```python
from build123d import *

# Parameters (mm, degrees)
SKETCH1_W                    = 42
SKETCH1_H                    = 42
SKETCH1_R                    = 1.65
SKETCH1_R_2                  = 18
BOSS_EXTRUDE1_DEPTH          = 13
CHAMFER1_SIZE                = 5.5
SKETCH3_R                    = 1.75
CUT_EXTRUDE2_DEPTH           = 20
SKETCH4_R                    = 1.75
CUT_EXTRUDE3_DEPTH           = 20
BOSS_EXTRUDE2_DEPTH          = 2
CUT_REVOLVE1_ANGLE           = 183.3
CUT_REVOLVE1_OTHER_WAY_ANGLE = 3.2


with BuildPart() as part:
    # Sketch1 → Boss-Extrude1 (new body)
    with BuildSketch(Plane(origin=(0, 0, 0), x_dir=(1, 0, 0), z_dir=(0, 1, 0))):
        with Locations((21, 21)):
            Rectangle(SKETCH1_W, SKETCH1_H)
        with Locations(Location((5.5, 36.5, 0), (0, 0, 90))):
            Circle(SKETCH1_R, mode=Mode.SUBTRACT)
        with Locations(Location((5.5, 5.5, 0), (0, 0, 90))):
            Circle(SKETCH1_R, mode=Mode.SUBTRACT)
        with Locations(Location((21, 21, 0), (0, 0, 90))):
            Circle(SKETCH1_R_2, mode=Mode.SUBTRACT)
    extrude(amount=BOSS_EXTRUDE1_DEPTH)

    # Chamfer1
    chamfer1_edges = [part.edges().sort_by_distance(p)[0] for p in [
        (0, 6.5, -42),
        (42, 6.5, -42),
        (42, 6.5, 0),
        (0, 6.5, 0),
    ]]
    chamfer(chamfer1_edges, length=CHAMFER1_SIZE)

    # Sketch3 → Cut-Extrude2 (cut)
    with BuildSketch(Plane(origin=(42, 0, 0), x_dir=(0, 0, -1), z_dir=(1, 0, 0))):
        with Locations(Location((37.4, 9, 0), (0, 0, 333.948601241))):
            Circle(SKETCH3_R)
    extrude(amount=-CUT_EXTRUDE2_DEPTH, mode=Mode.SUBTRACT)

    # Sketch4 → Cut-Extrude3 (cut)
    with BuildSketch(Plane(origin=(42, 0, 0), x_dir=(0, 0, -1), z_dir=(1, 0, 0))):
        with Locations(Location((4.6, 9, 0), (0, 0, 300.949723079))):
            Circle(SKETCH4_R)
    extrude(amount=-CUT_EXTRUDE3_DEPTH, mode=Mode.SUBTRACT)

    # Sketch6 → Boss-Extrude2 (add)
    with BuildSketch(Plane(origin=(0, 0, -42), x_dir=(-1, 0, 0), z_dir=(0, 0, -1))):
        Polygon((-23.468351512, 0.829629357), (-18.531648488, 0.829629357), (-18.531648488, 5.944922789), (-14.8, 5.944922789), (-21, 12.144922789), (-27.2, 5.944922789), (-23.468351512, 5.944922789), align=None)
    extrude(amount=BOSS_EXTRUDE2_DEPTH)

    # Sketch9 → Cut-Revolve1 (revolve, cut)
    with BuildSketch(Plane(origin=(21, 0, 0), x_dir=(0, 0, -1), z_dir=(1, 0, 0))):
        with BuildLine():
            Line((3.027799244, 9.768560202), (3.027799244, 8.231439798))
            ThreePointArc((3.027799244, 8.231439798), (2.85, 9), (3.027799244, 9.768560202))
        make_face()
    revolve(axis=Axis((21, 18.192178388, -21), (0, -1, 0)), revolution_arc=CUT_REVOLVE1_ANGLE, mode=Mode.SUBTRACT)

    # Sketch9 → Cut-Revolve1 other way (revolve, cut)
    with BuildSketch(Plane(origin=(21, 0, 0), x_dir=(0, 0, -1), z_dir=(1, 0, 0))):
        with BuildLine():
            Line((3.027799244, 9.768560202), (3.027799244, 8.231439798))
            ThreePointArc((3.027799244, 8.231439798), (2.85, 9), (3.027799244, 9.768560202))
        make_face()
    revolve(axis=Axis((21, 18.192178388, -21), (0, 1, 0)), revolution_arc=CUT_REVOLVE1_OTHER_WAY_ANGLE, mode=Mode.SUBTRACT)


solid = part.part
```
For this review, take the finished solid that the model builds, in its own axes (mm). A direction names the side the tool comes from. Give positions to 0.01 mm unless a question says otherwise; leave off trailing zeros. Write each loop counter-clockwise with the first axis right and the second up, starting at its lowest first coordinate (ties: lowest second). Pieces come first, ordered by that corner, then holes.
Item 1: Machinability: for faces 4 (the face through (24.057, 9.088, -42.986)), 5 (the face through (17.857, 9.002, -42.986)), 6 (the face through (34.36, 9.64, -2.97)), which of the approach directions +Z, -Z, +X, -X, +Y, -Y give a long, thin tool a straight path to every point of the face, cutting with its end or side? Answer none if there is none.
Item 2: Insertion check: P1, Ø1, axis at x = 21, z = -43, coming from the -Y side; P2, Ø1, axis at y = 3, z = -43.5, coming from the +X side; P3, Ø0.6, axis at x = 17.5, z = -43.5, coming from the -Y side; P4, Ø3, axis at x = 5.5, z = -5.5, coming from the +Y side. Each pin has a flat end and moves straight along its axis. Give the tip position at first contact, or say it passes through.
Item 3: Take a section at A-A (y = 9). Give the number of separate pieces and of enclosed holes in the cut face, and give its area (3 significant figures).
Item 4: Take a section at C-C (y = 1.75). Give the boundary of the cut face in (x, z), and give its area (3 significant figures).
Item 5: Take a section at D-D (x = 24). Give the boundary of the cut face in (y, z).
Item 6: Wall thickness on probe 1 along Z at (x, y) = (22, 3.75); probe 2 along X at (y, z) = (7, -36.5); probe 3 along Z at (x, y) = (36, 9): over which ranges is each line inside the solid? List them lowest first.
Item 7: The part is to be moulded in two halves that separate along X. For faces 1 (the face through (25, 5.945, -43)), 2 (the face through (23.468, 3, -43)), 3 (the face through (31.953, 6.409, -6.716)), say which applies: +X half, -X half, draft (parallel to the pull), parting line (faces both ways), or undercut.
Item 8: Take a section at B-B (z = -21). Give the boundary of the cut face in (x, y).
Established:
1. face 4: -Z, +X, +Y
1. face 5: -Z, -X, +Y
1. face 6: +X
2. P1: stops at y = 0.83
2. P2: stops at x = 23.47
2. P3: stops at y = 5.94
2. P4: passes through
3. separate pieces: 2
3. enclosed holes: 2
3. area: 580 mm2
4. outline: (0, -36.5) - (5.5, -42) - (18.53, -42) - (18.53, -44) - (23.47, -44) - (23.47, -42) - (36.5, -42) - (42, -36.5) - (42, -5.5) - (36.5, 0) - (5.5, 0) - (0, -5.5) - close; hole circle Ø36 at (21, -21); hole circle Ø3.3 at (5.5, -36.5); hole circle Ø3.3 at (5.5, -5.5)
4. area: 678 mm2
5. outline: (0, -42) - (5.94, -42) - (5.94, -44) - (9.14, -44) - (9.14, -42) - (13, -42) - (13, -38.75) - (10.12, -38.75) arc R1.75 cw to (7.88, -38.75) - (0, -38.75) - close; (0, -3.25) - (7.88, -3.25) arc R1.75 cw to (10.12, -3.25) - (13, -3.25) - (13, 0) - (0, 0) - close
6. probe 1: z = -44 to -38.97, -3.03 to 0
6. probe 2: x = 0 to 3.85, 7.15 to 11.85, 30.15 to 42
6. probe 3: z = -42 to -39.15, -35.65 to -30.95, -11.05 to -6.35, -2.85 to 0
7. face 1: draft
7. face 2: +X half
7. face 3: undercut
8. outline: (0, 0) - (3, 0) - (3, 8.29) arc R1.75 cw to (3, 9.71) - (3, 13) - (0, 13) - close; (39, 0) - (42, 0) - (42, 13) - (39, 13) - close
